```python
from build123d import *

# Parameters (mm, degrees)
F2_DEPTH = 22.86
F0_W     = 76.2
F0_H     = 23.8252
F3_DEPTH = 12.954
F4_W     = 19.05
F4_H     = 13.8684
F5_DEPTH = 74.422


with BuildPart() as f2:
    # F1 (on Top) → F2 (new body)
    with BuildSketch(Plane.XY):
        Polygon((-47.205903, 57.15), (-47.205903, 0), (29.019497, 0), (29.019497, 57.15), (5.194297, 57.15), (5.194297, 28.575), (-23.380703, 28.575), (-23.380703, 57.15), align=None)
    extrude(amount=-F2_DEPTH)

    # F0 (on Front) → F3 (join)
    with BuildSketch(Plane.XZ):
        with Locations((-8.839202, -34.4932)):
            Rectangle(F0_W, F0_H)
    extrude(amount=-F3_DEPTH)

    # F4 (on face) → F5 (join)
    with BuildSketch(Plane(origin=(-46.939202, 0, 0), x_dir=(0, -1, 0), z_dir=(-1, 0, 0))):
        with Locations((-9.525, 6.9342)):
            Rectangle(F4_W, F4_H)
    extrude(amount=-F5_DEPTH)


solid = f2.part
```
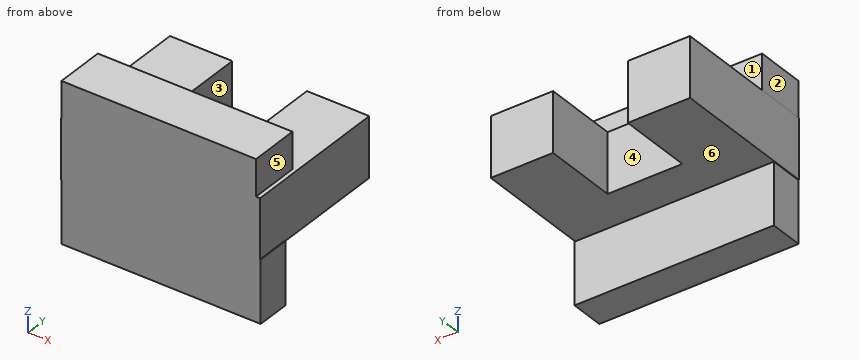
The listing builds one solid part. Answer for the finished solid, in the listing's coordinates (mm). Face numbers are marked on the shaded views. A direction names the side the tool comes from. Give positions to 0.01 mm unless a question says otherwise; leave off trailing zeros. Order: outer loops, then holes, each group sorted by start corner. A loop starts at its lowest first (then second) coordinate and runs counter-clockwise, first axis right, second up. Notation, with made-up numbers: (13.25, -5.5) - (44.25, -5.5) arc R24 ccw to (44.25, 32.5) - close; hole circle Ø2 at (50.25, 37). An arc over 180 degrees is marked (long way). Use one line per item in the form item = value. Start each with the question number.
(1) A cutting plane is placed at A-A, the plane y = 46. Write down the section's boundary in (x, z), then the cut area to 3 significant figures.
(2) The mould has two halves that part along X. Classify the marked faces 4, 5 and 6: released by +X, released by -X, zero draft, split by the parting line, or undercut.
(3) A cutting plane is placed at D-D, the plane y = 24.5. Write down the section's boundary in (x, z), then the cut area to 3 significant figures.
(4) Flat-ended cylindrical pins translate along their axes: pin 1 Ø15.5 at (y, z) = (5, 5.5) entering from +X; pin 2 Ø7 at (x, z) = (-13.5, -11) entering from +Y (3 decimals); pin 3 Ø5 at (x, y) = (-25, 46) entering from +Z; pin 4 Ø17 at (x, y) = (-9, 40) entering from +Z. Find the tip coordinate at first contact, or state that the pin passes through.
(5) Consider line 1 (Z direction, x = 21, y = 18.5); line 2 (Z direction, x = -21.5, y = 25); line 3 (X direction, y = 12, z = -25). Determine where each line is inside the solid, lowest interval first. Write a range as from..to.
(6) For the marked faces 1, 2 and 3, determine the directions among +Z, -Z, +X, -X, +Y, -Y from which every point of the face is accessible in a straight line to the end or side of a thin tool.
(7) A cutting plane is placed at B-B, the plane x = -10.5. Write down the section's boundary in (y, z) (3 decimals).
Ans:
q1.outline = (-47.21, -22.86) - (-23.38, -22.86) - (-23.38, 0) - (-47.21, 0) - close; (5.19, -22.86) - (29.02, -22.86) - (29.02, 0) - (5.19, 0) - close
q1.area = 1,090 mm^2
q2.face_4 = undercut
q2.face_5 = released by +X
q2.face_6 = zero draft
q3.outline = (-47.21, -22.86) - (29.02, -22.86) - (29.02, 0) - (-47.21, 0) - close
q3.area = 1,740 mm^2
q4.pin_1 = 29.02
q4.pin_2 = 28.575
q4.pin_3 = 0
q4.pin_4 = through
q5.line_1 = -22.86..13.87
q5.line_2 = -22.86..0
q5.line_3 = -46.94..29.26
q6.face_1 = +Z, +X, -X, +Y
q6.face_2 = +Z, -X, +Y, -Y
q6.face_3 = +Z, -Z, +Y
q7.outline = (0, -46.406) - (12.954, -46.406) - (12.954, -22.86) - (28.575, -22.86) - (28.575, 0) - (19.05, 0) - (19.05, 13.868) - (0, 13.868) - close
